```python
from build123d import *

# Parameters (mm, degrees)
SKETCH1_W           = 110
SKETCH1_H           = 40
BOSS_EXTRUDE1_DEPTH = 3
BOSS_EXTRUDE2_DEPTH = 3
SKETCH3_R           = 1
CUT_EXTRUDE1_DEPTH  = 3
SKETCH4_W           = 8
SKETCH4_H           = 3
SKETCH4_W_2         = 2.4
SKETCH4_H_2         = 6
CUT_EXTRUDE2_DEPTH  = 3
FILLET6_R           = 1
SKETCH5_W           = 8
SKETCH5_H           = 3
CUT_EXTRUDE3_DEPTH  = 10
FILLET7_R           = 1
SKETCH6_R           = 1.25
CUT_EXTRUDE4_DEPTH  = 62.424750712
SKETCH7_R           = 5
CUT_EXTRUDE5_DEPTH  = 10


with BuildPart() as part:
    # Sketch1 → Boss-Extrude1 (new body)
    with BuildSketch(Plane.XY):
        Rectangle(SKETCH1_W, SKETCH1_H)
    extrude(amount=BOSS_EXTRUDE1_DEPTH)

    # Sketch2 → Boss-Extrude2 (add)
    with BuildSketch(Plane.XY.offset(3)):
        Polygon((58, 10), (58, 13.5), (55, 13.5), (55, 6.5), (58, 6.5), align=None)
        Polygon((55, -10), (55, -6.5), (58, -6.5), (58, -13.5), (55, -13.5), align=None)
        Polygon((-55, 6.5), (-55, 13.5), (-58, 13.5), (-58, 10), (-58, 6.5), align=None)
        Polygon((-55, -13.5), (-55, -10), (-55, -6.5), (-58, -6.5), (-58, -13.5), align=None)
    extrude(amount=-BOSS_EXTRUDE2_DEPTH)

    # Sketch3 → Cut-Extrude1 (cut)
    with BuildSketch(Plane.XY.offset(3)):
        with Locations((-55, 14.5)):
            Circle(SKETCH3_R)
        with Locations((-55, 5.5)):
            Circle(SKETCH3_R)
        with Locations((-55, -5.5)):
            Circle(SKETCH3_R)
        with Locations((-55, -14.5)):
            Circle(SKETCH3_R)
        with Locations((55, 14.5)):
            Circle(SKETCH3_R)
        with Locations((55, 5.5)):
            Circle(SKETCH3_R)
        with Locations((55, -5.5)):
            Circle(SKETCH3_R)
        with Locations((55, -14.5)):
            Circle(SKETCH3_R)
    extrude(amount=-CUT_EXTRUDE1_DEPTH, mode=Mode.SUBTRACT)

    # Sketch4 → Cut-Extrude2 (cut)
    with BuildSketch(Plane.XY.offset(3)):
        with Locations((-51, 0)):
            Rectangle(SKETCH4_W, SKETCH4_H)
        Polygon((-47, 3), (-47, 1.5), (-47, -1.5), (-47, -3), (-44.6, -3), (-44.6, -1.5), (-44.6, 1.5), (-44.6, 3), align=None)
        with BuildLine():
            ThreePointArc((-44.6, -1.5), (-43.1, 0), (-44.6, 1.5))
            Line((-44.6, 1.5), (-44.6, -1.5))
        make_face()
        with Locations((45.8, 0)):
            Rectangle(SKETCH4_W_2, SKETCH4_H_2)
        with BuildLine():
            Line((44.6, -1.5), (44.6, 1.5))
            ThreePointArc((44.6, 1.5), (43.1, 0), (44.6, -1.5))
        make_face()
        with Locations((51, 0)):
            Rectangle(SKETCH4_W, SKETCH4_H)
    extrude(amount=-CUT_EXTRUDE2_DEPTH, mode=Mode.SUBTRACT)

    # Fillet6
    fillet6_edges = [part.edges().sort_by_distance(p)[0] for p in [
        (-47, 3, 1.5),
        (-44.6, 3, 1.5),
        (-44.6, -3, 1.5),
        (-47, -3, 1.5),
        (47, 3, 1.5),
        (47, -3, 1.5),
        (44.6, -3, 1.5),
        (44.6, 3, 1.5),
    ]]
    fillet(fillet6_edges, radius=FILLET6_R)

    # Sketch5 → Cut-Extrude3 (cut)
    with BuildSketch(Plane.XY.offset(3)):
        with Locations((-27.5, 0)):
            Rectangle(SKETCH5_W, SKETCH5_H)
        with Locations((27.5, 0)):
            Rectangle(SKETCH5_W, SKETCH5_H)
    extrude(amount=-CUT_EXTRUDE3_DEPTH, mode=Mode.SUBTRACT)

    # Fillet7
    fillet7_edges = [part.edges().sort_by_distance(p)[0] for p in [
        (-23.5, 1.5, 1.5),
        (-23.5, -1.5, 1.5),
        (-31.5, -1.5, 1.5),
        (-31.5, 1.5, 1.5),
        (31.5, 1.5, 1.5),
        (31.5, -1.5, 1.5),
        (23.5, -1.5, 1.5),
        (23.5, 1.5, 1.5),
    ]]
    fillet(fillet7_edges, radius=FILLET7_R)

    # Sketch6 → Cut-Extrude4 (cut, through all)
    with BuildSketch(Plane.XY.offset(3)):
        with Locations((-40, -14)):
            Circle(SKETCH6_R)
        with Locations((-20, -14)):
            Circle(SKETCH6_R)
        with Locations((0, -14)):
            Circle(SKETCH6_R)
        with Locations((20, -14)):
            Circle(SKETCH6_R)
        with Locations((40, -14)):
            Circle(SKETCH6_R)
        with Locations((40, 14)):
            Circle(SKETCH6_R)
        with Locations((20, 14)):
            Circle(SKETCH6_R)
        with Locations((0, 14)):
            Circle(SKETCH6_R)
        with Locations((-20, 14)):
            Circle(SKETCH6_R)
        with Locations((-40, 14)):
            Circle(SKETCH6_R)
    extrude(amount=-CUT_EXTRUDE4_DEPTH, mode=Mode.SUBTRACT)

    # Sketch7 → Cut-Extrude5 (cut)
    with BuildSketch(Plane.XY.offset(3)):
        with Locations((-40, 12.75)):
            Circle(SKETCH7_R)
        with Locations((-40, -12.75)):
            Circle(SKETCH7_R)
        with Locations((40, 12.75)):
            Circle(SKETCH7_R)
        with Locations((40, -12.75)):
            Circle(SKETCH7_R)
    extrude(amount=-CUT_EXTRUDE5_DEPTH, mode=Mode.SUBTRACT)


solid = part.part
```
The model under review builds one solid part; all positions refer to its coordinate system, in mm. A direction names the side the tool comes from. Round coordinates to 2 decimals unless told otherwise and drop trailing zeros. Write each loop counter-clockwise with the first axis right and the second up, starting at its lowest first coordinate (ties: lowest second). Pieces come first, ordered by that corner, then holes. Notation, with made-up numbers: M 43.5,59 L 90.5,59 A16 cw 90.5,88 Z; hole C -1,83 d9. An arc over 180 degrees is marked long. Use CSV: the item, a comma, the result in double quotes. Start each with the question number.
(1) We need section A-A, the plane x = 48. State the section outline as (y, z) points, then the cut area to 3 significant figures.
(2) The part is to be moulded in two halves that separate along X. For faces 6 (the face through (57, 13.5, 2)), 7 (the face through (20.672, -12.946, 1.521)), 8 (the face through (55, -3, 1)), say which applies: +X half, -X half, draft (parallel to the pull), parting line (faces both ways), or undercut.
(3) Tool access review of faces 1 (the face through (-56, 13.5, 2)), 2 (the face through (55, -18, 1)), 3 (the face through (-57, 6.5, 2)), 4 (the face through (-28, 1.5, 2)), 5 (the face through (56, -6.5, 2)): name each direction out of +Z, -Z, +X, -X, +Y, -Y from which nothing blocks a thin tool from reaching the whole face with its end or side.
(4) For line 1 along Y through (x, z) = (-20, 2.15); line 2 along Y through (x, z) = (40, 1.6); line 3 along Y through (x, z) = (-28, 2.3), list the stretches that pass through material, from the lowest coordinate up.
(5) We need section C-C, the plane x = -40. State the section outline as (y, z) points.
(6) Clearance check with flat-ended pins moving along their axes: P1, Ø11.5, axis at x = -40, y = 12.75, coming from the +Z side; P2, Ø2, axis at x = 0, y = 14, coming from the +Z side; P3, Ø0.9, axis at x = 57, z = 1, coming from the -Y side; P4, Ø0.8, axis at y = 0, z = 2, coming from the -X side. State where each tip first meets the part, or that it passes through.
(7) We need section D-D, the plane z = 1.7. State how many separate pieces and enclosed holes the cut face has, then the cut area to 3 significant figures.
(8) We need section B-B, the plane x = -20. State the section outline as (y, z) points.
Findings:
1,outline,"M -20,0 L -1.5,0 L -1.5,3 L -20,3 Z; M 1.5,0 L 20,0 L 20,3 L 1.5,3 Z"
1,area,"111 mm^2"
2,face 6,"draft"
2,face 7,"undercut"
2,face 8,"+X half"
3,face 1,"+Z, -Z, -X, +Y"
3,face 2,"+Z, -Z, +X, -Y"
3,face 3,"+Z, -Z, -X"
3,face 4,"+Z, -Z"
3,face 5,"+Z, -Z, +X"
4,line 1,"-20 to -15.25, -12.75 to 12.75, 15.25 to 20"
4,line 2,"-20 to -17.75, -7.75 to 7.75, 17.75 to 20"
4,line 3,"-20 to -1.5, 1.5 to 20"
5,outline,"M -20,0 L -17.75,0 L -17.75,3 L -20,3 Z; M -7.75,0 L 7.75,0 L 7.75,3 L -7.75,3 Z; M 17.75,0 L 20,0 L 20,3 L 17.75,3 Z"
6,P1,"z = 3"
6,P2,"through"
6,P3,"y = -13.5"
6,P4,"x = -43.15"
7,separate pieces,"1"
7,enclosed holes,"12"
7,area,"4,000 mm^2"
8,outline,"M -20,0 L -15.25,0 L -15.25,3 L -20,3 Z; M -12.75,0 L 12.75,0 L 12.75,3 L -12.75,3 Z; M 15.25,0 L 20,0 L 20,3 L 15.25,3 Z"
